Can you work these out from the drawing? Everything is in mm from the part's minimum corner. Coordinates: 2 decimals unless noted, no trailing zeros. Order: outer loops, then holes, each group sorted by start corner. A loop starts at its lowest first (then second) coordinate and runs counter-clockwise, first axis right, second up. Notation, with made-up numbers: (81.5, 58.25) - (97.5, 58.25) arc R22 ccw to (97.5, 66.25) - close; hole circle Ø3 at (9, 10). An arc over 180 degrees is marked (long way). One line per item, written item: value.
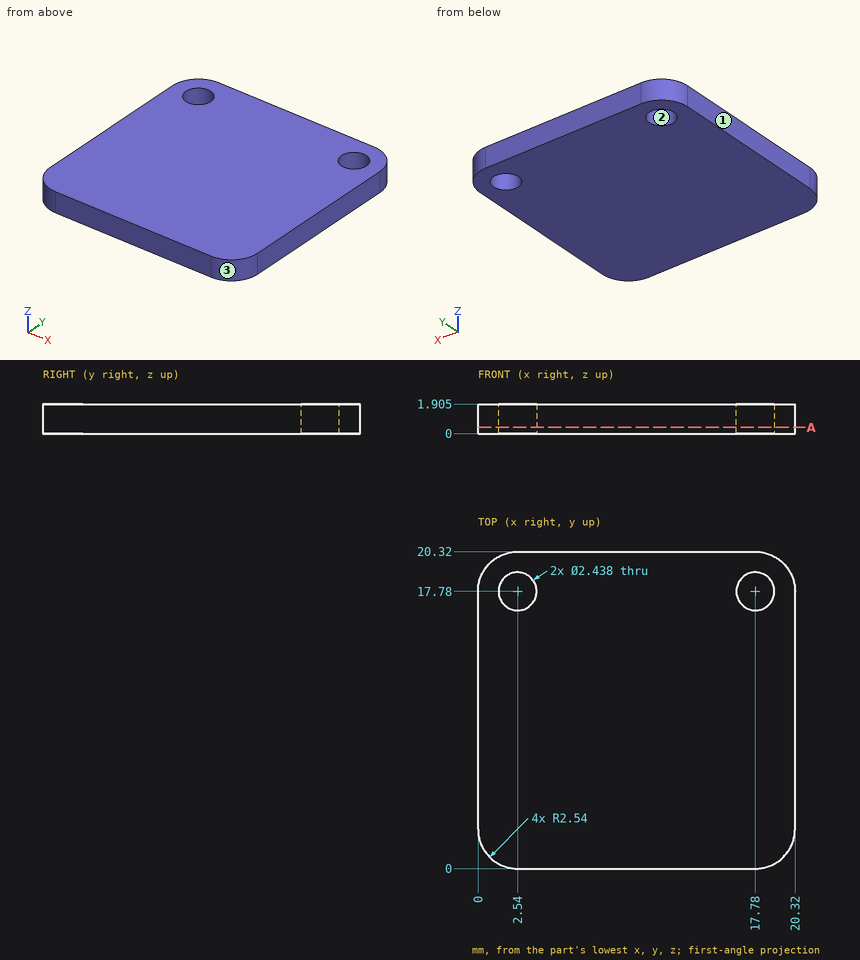
Item 1: If I drill on probe 1 along Y at (x, z) = (17.78, 1.3); probe 2 along Y at (x, z) = (17, 0.95) (1 decimal); probe 3 along X at (y, z) = (1.5, 0.45), over which ranges is the centre line in solid material (lowest first)?
Conclusion:
probe 1: 0 to 16.56, 19 to 20.32
probe 2: 0 to 16.8, 18.7 to 20.3
probe 3: 0.22 to 20.1
Item 2: I want a section at A-A on z = 0.4. Please give me the cut outline in (x, y).
Conclusion:
outline: (0, 2.54) arc R2.54 ccw to (2.54, 0) - (17.78, 0) arc R2.54 ccw to (20.32, 2.54) - (20.32, 17.78) arc R2.54 ccw to (17.78, 20.32) - (2.54, 20.32) arc R2.54 ccw to (0, 17.78) - close; hole circle Ø2.44 at (2.54, 17.78); hole circle Ø2.44 at (17.78, 17.78)
Item 3: I'm going to push a flat-ended pin straight in: pin 1 Ø2 at (x, y) = (2.54, 17.78) entering from +Z. Where does the tip first touch, or does it pass through?
Conclusion:
pin 1: through
Item 4: Thinking about a two-plate mould opening in Y: for the marked faces 1, 2 and 3, which applies, pulls with the +Y half, pulls with the -Y half, needs draft (parallel to the pull), parting line crosses it, or undercut?
Conclusion:
face 1: needs draft
face 2: undercut
face 3: pulls with the -Y half
